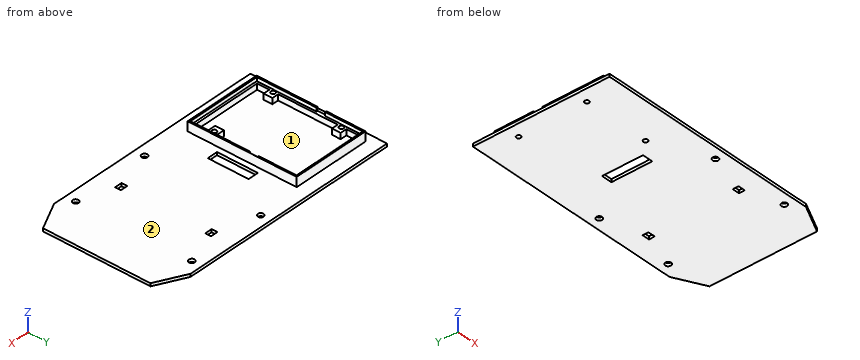
```python
from build123d import *

# Parameters (mm, degrees)
PAD_DEPTH       = 2
SKETCH001_W     = 54
SKETCH001_H     = 75
PAD001_DEPTH    = 4
SKETCH002_W     = 54
SKETCH002_H     = 75
SKETCH002_W_2   = 52
SKETCH002_H_2   = 73
PAD002_DEPTH    = 2.5
SKETCH003_R     = 1.5
POCKET_DEPTH    = 6.001
SKETCH004_W     = 1.028311
SKETCH004_H     = 6
SKETCH004_W_2   = 1.0671
POCKET001_DEPTH = 2.5
SKETCH005_W     = 5
SKETCH005_H     = 4
POCKET002_DEPTH = 2.001
SKETCH006_R     = 2
POCKET003_DEPTH = 2.001
SKETCH007_W     = 7.274784
SKETCH007_H     = 28.1615223689
POCKET004_DEPTH = 5


with BuildPart() as part:
    # Sketch → Pad (new body)
    with BuildSketch(Plane.XY):
        Polygon((-26, 47), (-26, -47), (128, -47), (148, -37), (148, 37), (128, 47), align=None)
    extrude(amount=PAD_DEPTH)

    # Sketch001 → Pad001 (new body)
    with BuildSketch(Plane.XY.offset(2)):
        with Locations((7, 0)):
            Rectangle(SKETCH001_W, SKETCH001_H)
        Polygon((-17.5, 35), (31.5, 35), (31.5, -20.5), (25, -20.5), (25, -26.5), (31.5, -26.5), (31.5, -35), (-17.5, -35), (-17.5, -26.5), (-13, -26.5), (-13, -20.5), (-17.5, -20.5), (-17.5, 20.5), (-13, 20.5), (-13, 26.5), (-17.5, 26.5), align=None, mode=Mode.SUBTRACT)
    extrude(amount=PAD001_DEPTH)

    # Sketch002 → Pad002 (new body)
    with BuildSketch(Plane.XY.offset(6)):
        with Locations((7, 0)):
            Rectangle(SKETCH002_W, SKETCH002_H)
        with Locations((7, 0)):
            Rectangle(SKETCH002_W_2, SKETCH002_H_2, mode=Mode.SUBTRACT)
    extrude(amount=PAD002_DEPTH)

    # Sketch003 → Pocket (cut, through all)
    with BuildSketch(Plane.XY.offset(6)):
        with Locations((-17, 23.5)):
            Circle(SKETCH003_R)
        with Locations((-17, -23.5)):
            Circle(SKETCH003_R)
        with Locations((29, -23.5)):
            Circle(SKETCH003_R)
    extrude(amount=-POCKET_DEPTH, mode=Mode.SUBTRACT)

    # Sketch004 → Pocket001 (cut)
    with BuildSketch(Plane.XY.offset(8.5)):
        with Locations((-19.4858445, 7.5)):
            Rectangle(SKETCH004_W, SKETCH004_H)
        with Locations((33.439625, 7.5)):
            Rectangle(SKETCH004_W_2, SKETCH004_H)
    extrude(amount=-POCKET001_DEPTH, mode=Mode.SUBTRACT)

    # Sketch005 → Pocket002 (cut, through all)
    with BuildSketch(Plane.XY.offset(2)):
        with Locations((93.5, 31)):
            Rectangle(SKETCH005_W, SKETCH005_H)
        with Locations((93.5, -31)):
            Rectangle(SKETCH005_W, SKETCH005_H)
    extrude(amount=-POCKET002_DEPTH, mode=Mode.SUBTRACT)

    # Sketch006 → Pocket003 (cut, through all)
    with BuildSketch(Plane.XY.offset(2)):
        with Locations((119, 40)):
            Circle(SKETCH006_R)
        with Locations((65, 40)):
            Circle(SKETCH006_R)
        with Locations((119, -40)):
            Circle(SKETCH006_R)
        with Locations((65, -40)):
            Circle(SKETCH006_R)
    extrude(amount=-POCKET003_DEPTH, mode=Mode.SUBTRACT)

    # Sketch007 → Pocket004 (cut)
    with BuildSketch(Plane.XY.offset(2)):
        with Locations((41.362608, 0)):
            Rectangle(SKETCH007_W, SKETCH007_H)
    extrude(amount=-POCKET004_DEPTH, mode=Mode.SUBTRACT)


solid = part.part
```
Geometry check sheet. Reference: the model listing, model coordinates, mm. Face numbers are marked on the shaded views. Give positions to 0.01 mm unless a question says otherwise; leave off trailing zeros. Loops run counter-clockwise (first coordinate to the right, second up) from the corner with the lowest first, then second, coordinate; pieces in that order, holes last. Notation, with made-up numbers: M -20,-30 L 31,-30 A21 cw 31,-20 Z; hole C -38,53.5 d8. An arc over 180 degrees is marked long. Write item = value, one per line. Start each with the question number.
1. Section check D-D, the plane x = 71. Enter the section's corners in (y, z), plus the area to 3 significant figures.
2. Go/stop test with flat-tipped pins: P1, Ø0.8, axis at y = 21, z = 7, coming from the +X side; P2, Ø1, axis at x = 63.5, y = 31, coming from the +Z side; P3, Ø4.5, axis at x = -14, z = 5, coming from the +Y side. Record where each tip stops, or that it passes through.
3. Section check A-A, the plane y = -7.5. Enter the section's corners in (x, z).
4. Thickness scan on probe 1 along Y at (x, z) = (119, 1.3); probe 2 along Y at (x, z) = (-17, 3.7); probe 3 along Y at (x, z) = (21.5, 4.5). Record the ranges inside material, lowest first.
5. Draft check along Y on the marked faces 1 and 2. Enter one of: +Y half, -Y half, draft (parallel to the pull), parting line (faces both ways), or undercut.
6. Section check B-B, the plane x = 119. Enter the section's corners in (y, z).
7. Section check C-C, the plane y = -40. Enter the section's corners in (x, z).
Values follow:
q1.outline = M -47,0 L 47,0 L 47,2 L -47,2 Z
q1.area = 188 mm^2
q2.P1 = 34
q2.P2 = 2
q2.P3 = 37.5
q3.outline = M -26,0 L 37.73,0 L 37.73,2 L 34,2 L 34,8.5 L 33,8.5 L 33,6 L 31.5,6 L 31.5,2 L -17.5,2 L -17.5,6 L -19,6 L -19,8.5 L -20,8.5 L -20,2 L -26,2 Z; M 45,0 L 148,0 L 148,2 L 45,2 Z
q4.probe_1 = -47 to -42, -38 to 38, 42 to 47
q4.probe_2 = -37.5 to -35, -26.5 to -25, -22 to -20.5, 20.5 to 22, 25 to 26.5, 35 to 37.5
q4.probe_3 = -37.5 to -35, 35 to 37.5
q5.face_1 = undercut
q5.face_2 = draft
q6.outline = M -47,0 L -42,0 L -42,2 L -47,2 Z; M -38,0 L 38,0 L 38,2 L -38,2 Z; M 42,0 L 47,0 L 47,2 L 42,2 Z
q7.outline = M -26,0 L 63,0 L 63,2 L -26,2 Z; M 67,0 L 117,0 L 117,2 L 67,2 Z; M 121,0 L 142,0 L 142,2 L 121,2 Z
